Input: part model. Units: mm. Frame: model coordinates. A direction names the side the tool comes from. Give positions to 0.01 mm unless a question says otherwise; leave off trailing zeros. Loops run counter-clockwise (first coordinate to the right, second up) from the corner with the lowest first, then second, coordinate; pieces in that order, holes last.
from build123d import *

# Parameters (mm, degrees)
BOSS_EXTRU_1_DEPTH      = 1980
ENL_V_MAT_EXTRU_1_DEPTH = 1981.194091497
ESQUISSE3_W             = 4.3
ESQUISSE3_H             = 0.35
ENL_V_MAT_EXTRU_2_DEPTH = 1980
ESQUISSE4_W             = 1.625
ESQUISSE4_H             = 14.5
ENL_V_MAT_EXTRU_3_DEPTH = 1981.194091497
ENL_V_MAT_EXTRU_4_DEPTH = 1981.194091497
D_POUILLE1_ANGLE        = 20
D_POUILLE2_ANGLE        = 20
D_POUILLE3_ANGLE        = 45
PER_AGE1_D              = 6
PER_AGE1_DEPTH          = 20
PER_AGE1_CBORE_D        = 9.5
PER_AGE1_CBORE_DEPTH    = 8.5
CHANFREIN1_SIZE         = 0.8
CHANFREIN2_SIZE         = 1.2
CHANFREIN2_SIZE2        = 0.692820323
CHANFREIN3_SIZE         = 0.2
CHANFREIN4_SIZE         = 0.692820323
CHANFREIN4_SIZE2        = 1.2
ENL_V_START             = -120
ESQUISSE12_W            = 78.153878041
ESQUISSE12_H            = 74.514600195
ENL_V_MAT_EXTRU_5_DEPTH = 1861.194091497


with BuildPart() as part:
    # Esquisse1 → Boss.-Extru.1 (new body)
    with BuildSketch(Plane(origin=(0, 0, 0), x_dir=(-1, 0, 0), z_dir=(0, 0, -1))):
        with BuildLine():
            Line((-19.2, 7.973691854), (-19.2, 0))
            Line((-19.2, 0), (0.8, 0))
            Line((0.8, 0), (0.8, 20))
            Line((0.8, 20), (-17.575, 20))
            Line((-17.575, 20), (-17.575, 17.767136655))
            ThreePointArc((-17.575, 17.767136655), (-16.197491801, 17.200016465), (-15.5625262, 15.852436102))
            Line((-15.5625262, 15.852436102), (-15.5625262, 9.147563898))
            ThreePointArc((-15.5625262, 9.147563898), (-16.984759825, 7.331984363), (-19.2, 7.973691854))
        make_face()
    extrude(amount=-BOSS_EXTRU_1_DEPTH)

    # Esquisse2 → Enlèv. mat.-Extru.1 (cut, through all)
    with BuildSketch(Plane.XY.offset(1980)):
        with BuildLine():
            Line((17.575, 7.232863345), (17.575, 4.908548369))
            Line((17.575, 4.908548369), (19.2, 4.908548369))
            Line((19.2, 4.908548369), (19.2, 7.973691854))
            ThreePointArc((19.2, 7.973691854), (18.471955551, 7.418025184), (17.575, 7.232863345))
        make_face()
    extrude(amount=-ENL_V_MAT_EXTRU_1_DEPTH, mode=Mode.SUBTRACT)

    # Esquisse3 → Enlèv. mat.-Extru.2 (cut)
    with BuildSketch(Plane.XY.offset(1980)):
        with Locations((9.2, 0.175)):
            Rectangle(ESQUISSE3_W, ESQUISSE3_H)
    extrude(amount=-ENL_V_MAT_EXTRU_2_DEPTH, mode=Mode.SUBTRACT)

    # Esquisse4 → Enlèv. mat.-Extru.3 (cut, through all)
    with BuildSketch(Plane.XY.offset(1980)):
        with Locations((0.0125, 12.75)):
            Rectangle(ESQUISSE4_W, ESQUISSE4_H)
    extrude(amount=-ENL_V_MAT_EXTRU_3_DEPTH, mode=Mode.SUBTRACT)

    # Esquisse5 → Enlèv. mat.-Extru.4 (cut, through all)
    with BuildSketch(Plane.XY.offset(1980)):
        with BuildLine():
            Line((0.825, 17.767136655), (0.825, 7.232863345))
            ThreePointArc((0.825, 7.232863345), (2.202508199, 7.799983535), (2.8374738, 9.147563898))
            Line((2.8374738, 9.147563898), (2.8374738, 15.852436102))
            ThreePointArc((2.8374738, 15.852436102), (2.202508199, 17.200016465), (0.825, 17.767136655))
        make_face()
    extrude(amount=-ENL_V_MAT_EXTRU_4_DEPTH, mode=Mode.SUBTRACT)

    # Dépouille1
    d_pouille1_faces = [part.faces().sort_by_distance(p)[0] for p in [
        (0.0125, 5.5, 990),
    ]]
    draft(d_pouille1_faces, Plane(origin=(0.825, 5.5, 0), x_dir=(0, -1, 0), z_dir=(-1, 0, 0)), D_POUILLE1_ANGLE)

    # Dépouille2
    d_pouille2_faces = [part.faces().sort_by_distance(p)[0] for p in [
        (18.3875, 4.908548369, 990),
    ]]
    draft(d_pouille2_faces, Plane(origin=(19.2, 7.973691854, 1980), x_dir=(0, 0, 1), z_dir=(1, 0, 0)), D_POUILLE2_ANGLE)

    # Dépouille3
    d_pouille3_faces = [part.faces().sort_by_distance(p)[0] for p in [
        (11.35, 0.175, 990),
        (7.05, 0.175, 990),
    ]]
    draft(d_pouille3_faces, Plane(origin=(11.35, 0.35, 0), x_dir=(0, 0, -1), z_dir=(0, -1, 0)), D_POUILLE3_ANGLE)

    # Perçage1
    with Locations(Plane(origin=(0, 20, 0), x_dir=(1, 0, 0), z_dir=(0, 1, 0))):
        with Locations((9.2, -30), (9.2, -90), (9.2, -150), (9.2, -210), (9.2, -270), (9.2, -330), (9.2, -390), (9.2, -450), (9.2, -510), (9.2, -570), (9.2, -630), (9.2, -690), (9.2, -750), (9.2, -810), (9.2, -870), (9.2, -930), (9.2, -990), (9.2, -1050), (9.2, -1110), (9.2, -1170), (9.2, -1230), (9.2, -1290), (9.2, -1350), (9.2, -1410), (9.2, -1470), (9.2, -1530), (9.2, -1590), (9.2, -1650), (9.2, -1710), (9.2, -1770), (9.2, -1830), (9.2, -1890), (9.2, -1950)):
            CounterBoreHole(PER_AGE1_D / 2, PER_AGE1_CBORE_D / 2, PER_AGE1_CBORE_DEPTH, depth=PER_AGE1_DEPTH)

    # Chanfrein1
    chanfrein1_edges = [part.edges().sort_by_distance(p)[0] for p in [
        (-0.8, 0, 990),
        (19.2, 0, 990),
    ]]
    chamfer(chanfrein1_edges, length=CHANFREIN1_SIZE)

    # Chanfrein2
    chanfrein2_edges = [part.edges().sort_by_distance(p)[0] for p in [
        (0.825, 20, 990),
    ]]
    chanfrein2_side = [part.faces().sort_by_distance(p)[0] for p in [
        (9.2, 20, 19.800708478),
    ]]
    chamfer(chanfrein2_edges, length=CHANFREIN2_SIZE, length2=CHANFREIN2_SIZE2, reference=chanfrein2_side[0])

    # Chanfrein3
    chanfrein3_edges = [part.edges().sort_by_distance(p)[0] for p in [
        (12.2, 0, 1950),
        (6.327718677, 0, 1949.133974596),
        (4.45, 20, 1950),
    ]]
    chamfer(chanfrein3_edges, length=CHANFREIN3_SIZE)

    # Chanfrein4
    chanfrein4_edges = [part.edges().sort_by_distance(p)[0] for p in [
        (17.575, 20, 990),
    ]]
    chanfrein4_side = [part.faces().sort_by_distance(p)[0] for p in [
        (17.575, 18.883568328, 990),
    ]]
    chamfer(chanfrein4_edges, length=CHANFREIN4_SIZE, length2=CHANFREIN4_SIZE2, reference=chanfrein4_side[0])

    # Esquisse12 → Enlèv. mat.-Extru.5 (cut, through all)
    with BuildSketch(Plane.XY.offset(1980).offset(ENL_V_START)):
        with Locations((15.863080013, 8.671326529)):
            Rectangle(ESQUISSE12_W, ESQUISSE12_H)
    extrude(amount=-ENL_V_MAT_EXTRU_5_DEPTH, mode=Mode.SUBTRACT)


solid = part.part
(1) Reachability of faces 4 (the cylindrical face through (8.58, 15.71, 1945.29)), 5 (the flat face through (9, 0.35, 1874)), 6 (the cylindrical face through (2.2, 17.2, 1920.8)) from +Z, -Z, +X, -X, +Y, -Y: full face, straight path, thin tool, end or side. Return the list, or none.
Values follow:
face 4: +Y
face 5: +Z, -Z, -Y
face 6: +Z, -Z, -X
(2) Pin query (flat end, axial travel): pin 1 Ø8.5 at (x, z) = (9.2, 1890) entering from +Y; pin 2 Ø0.5 at (y, z) = (18.5, 1914.5) entering from +X (3 decimals); pin 3 Ø3.5 at (x, z) = (9, 1869.5) entering from -Y. Return the tip coordinate at first contact, or that it passes through.
Values follow:
pin 1: stops at y = 11.5
pin 2: stops at x = 17.575
pin 3: stops at y = 0.35
(3) Cut plane B-B (x = 9.2). Return the cut outline in (y, z), and give its area (3 significant figures).
Values follow:
outline: (0.35, 1860) - (20, 1860) - (20, 1885.25) - (11.5, 1885.25) - (11.5, 1887) - (0.35, 1887) - close; (0.35, 1893) - (11.5, 1893) - (11.5, 1894.75) - (20, 1894.75) - (20, 1945.05) - (19.8, 1945.25) - (11.5, 1945.25) - (11.5, 1947) - (0.35, 1947) - close; (0.35, 1953) - (11.5, 1953) - (11.5, 1954.75) - (19.8, 1954.75) - (20, 1954.95) - (20, 1980) - (0.35, 1980) - close
area: 2,060 mm2
(4) Ray query, probe 1 along Z at (x, y) = (9.2, 15); probe 2 along Z at (x, y) = (9.2, 9); probe 3 along X at (y, z) = (4.25, 1950). Return the intervals inside material, ascending.
Values follow:
probe 1: z = 1860 to 1885.25, 1894.75 to 1945.25, 1954.75 to 1980
probe 2: z = 1860 to 1887, 1893 to 1947, 1953 to 1980
probe 3: x = -0.8 to 6.2, 12.2 to 19.2
(5) Cut plane A-A (z = 1890). Return the cut outline in (x, y) (3 decimals), and give its area (3 significant figures).
Values follow:
outline: (-0.8, 0.8) - (0, 0) - (6.2, 0) - (6.2, 11.5) - (4.45, 11.5) - (4.45, 20) - (2.025, 20) - (0.825, 19.307) - (0.825, 17.767) arc R2.06 cw to (2.837, 15.852) - (2.837, 9.148) arc R2.06 cw to (0.825, 7.233) - (0.825, 5.5) - (-0.8, 4.909) - close; (12.2, 0) - (18.4, 0) - (19.2, 0.8) - (19.2, 4.909) - (17.575, 5.5) - (17.575, 7.233) arc R2.06 cw to (15.563, 9.148) - (15.563, 15.852) arc R2.06 cw to (17.575, 17.767) - (17.575, 19.307) - (16.375, 20) - (13.95, 20) - (13.95, 11.5) - (12.2, 11.5) - close
area: 162 mm2
(6) Mould query, pull axis X, two halves, no side actions, for faces 1 (the flat face through (10.2, 11.5, 1953.1)), 2 (the flat face through (9, 10, 1980)), 3 (the cylindrical face through (2.2, 7.8, 1920.8)). Classes: +X half, -X half, draft (parallel to the pull), parting line (faces both ways), or undercut.
Values follow:
face 1: undercut
face 2: draft
face 3: -X half
